from build123d import *

# Parameters (mm, degrees)
SKETCH1_W           = 210
SKETCH1_H           = 270
SKETCH1_R           = 7.75
BOSS_EXTRUDE2_DEPTH = 6
CUT_EXTRUDE1_DEPTH  = 10
SKETCH4_R           = 1.25
CUT_EXTRUDE2_DEPTH  = 10
SKETCH5_R           = 6
CUT_EXTRUDE3_DEPTH  = 10


with BuildPart() as part:
    # Sketch1 → Boss-Extrude2 (new body)
    with BuildSketch(Plane(origin=(0, 0, 0), x_dir=(1, 0, 0), z_dir=(0, 1, 0))):
        with Locations((0, -10)):
            Rectangle(SKETCH1_W, SKETCH1_H)
        with Locations(Location((0, 0, 0), (0, 0, 270))):
            Circle(SKETCH1_R, mode=Mode.SUBTRACT)
    extrude(amount=BOSS_EXTRUDE2_DEPTH)

    # Sketch3 → Cut-Extrude1 (cut)
    with BuildSketch(Plane.XZ):
        with BuildLine():
            Line((17.000022153, 29.5), (17.000022153, 29.4))
            ThreePointArc((17.000022153, 29.4), (15.500022153, 27.9), (14.000022153, 29.4))
            Line((14.000022153, 29.4), (14.000022153, 29.5))
            ThreePointArc((14.000022153, 29.5), (15.500022153, 31), (17.000022153, 29.5))
        make_face()
        with BuildLine():
            Line((17.000022153, 60.5), (17.000022153, 60.4))
            ThreePointArc((17.000022153, 60.4), (15.500022153, 58.9), (14.000022153, 60.4))
            Line((14.000022153, 60.4), (14.000022153, 60.5))
            ThreePointArc((14.000022153, 60.5), (15.500022153, 62), (17.000022153, 60.5))
        make_face()
        with BuildLine():
            Line((-16.999993108, 29.500016738), (-16.999993206, 29.400016738))
            ThreePointArc((-16.999993206, 29.400016738), (-15.499994683, 27.900015261), (-13.999993206, 29.400013784))
            Line((-13.999993206, 29.400013784), (-13.999993108, 29.500013784))
            ThreePointArc((-13.999993108, 29.500013784), (-15.499991631, 31.000015261), (-16.999993108, 29.500016738))
        make_face()
        with BuildLine():
            Line((-16.999962586, 60.500016738), (-16.999962684, 60.400016738))
            ThreePointArc((-16.999962684, 60.400016738), (-15.499964161, 58.900015261), (-13.999962684, 60.400013784))
            Line((-13.999962684, 60.400013784), (-13.999962586, 60.500013784))
            ThreePointArc((-13.999962586, 60.500013784), (-15.499961109, 62.000015261), (-16.999962586, 60.500016738))
        make_face()
        with BuildLine():
            Line((11.250022153, 44.999994462), (11.250022104, 44.899994462))
            ThreePointArc((11.250022104, 44.899994462), (1.6566e-05, 33.65), (-11.249977896, 44.900005538))
            Line((-11.249977896, 44.900005538), (-11.249977847, 45.000005538))
            ThreePointArc((-11.249977847, 45.000005538), (2.7692e-05, 56.25), (11.250022153, 44.999994462))
        make_face()
    extrude(amount=-CUT_EXTRUDE1_DEPTH, mode=Mode.SUBTRACT)

    # Sketch4 → Cut-Extrude2 (cut)
    with BuildSketch(Plane.XZ):
        with Locations(Location((49.170333674, -115.382230576, 0), (0, 0, 270))):
            Circle(SKETCH4_R)
        with Locations(Location((-44.829666326, -115.382230576, 0), (0, 0, 270))):
            Circle(SKETCH4_R)
        with Locations(Location((49.170333674, -40.382230576, 0), (0, 0, 270))):
            Circle(SKETCH4_R)
        with Locations(Location((-44.829666326, -40.382230576, 0), (0, 0, 270))):
            Circle(SKETCH4_R)
    extrude(amount=-CUT_EXTRUDE2_DEPTH, mode=Mode.SUBTRACT)

    # Sketch5 → Cut-Extrude3 (cut)
    with BuildSketch(Plane(origin=(0, 6, 0), x_dir=(1, 0, 0), z_dir=(0, 1, 0))):
        with Locations(Location((-11.927460167, -114.387337557, 0), (0, 0, 270))):
            Circle(SKETCH5_R)
    extrude(amount=-CUT_EXTRUDE3_DEPTH, mode=Mode.SUBTRACT)


solid = part.part
Input: part model. Units: mm. Frame: model coordinates. Coordinates: 2 decimals unless noted, no trailing zeros. Order: outer loops, then holes, each group sorted by start corner. A loop starts at its lowest first (then second) coordinate and runs counter-clockwise, first axis right, second up. Notation, with made-up numbers: M 49,2 L 53,2 A25 cw 53,39 Z; hole C -34.75,83 d1. An arc over 180 degrees is marked long. One line per question, with ' | ' between items.
Item 1: Ray query, line 1 along Z through (x, y) = (49, 1.4); line 2 along X through (y, z) = (1.5, 0); line 3 along X through (y, z) = (4.55, -41). Return the intervals inside material, ascending.
Geometry results:
line 1: z = -125 to -116.62, -114.14 to -41.62, -39.14 to 145 | line 2: x = -105 to -7.75, 7.75 to 105 | line 3: x = -105 to -45.92, -43.74 to 48.08, 50.26 to 105
Item 2: Section A-A (z = 0). Output: boundary loops of the cut face in (x, y), then the cut area to 3 significant figures.
Geometry results:
outline: M -105,0 L -7.75,0 L -7.75,6 L -105,6 Z; M 7.75,0 L 105,0 L 105,6 L 7.75,6 Z | area: 1,170 mm^2
Item 3: Draft query along Z for faces 1 (the flat face through (105, 3, 12)), 2 (the flat face through (-1, 3, 145)), 3 (the cylindrical face through (-0.247, 2.958, 56.247)), 4 (the cylindrical face through (0.247, 2.958, 33.653)). Return one class per face: released by +Z, released by -Z, zero draft, split by the parting line, or undercut.
Geometry results:
face 1: zero draft | face 2: released by +Z | face 3: undercut | face 4: undercut
Item 4: Pin query (flat end, axial travel): pin 1 (4 mm diameter, centred on x = -44.83, z = -115.38, fed in from -Y). Return the tip coordinate at first contact, or that it passes through.
Geometry results:
pin 1: stops at y = 0
